CAD build for the part. Positions are in the model's coordinates, mm. A direction names the side the tool comes from. Coordinates: 2 decimals unless noted, no trailing zeros. Order: outer loops, then holes, each group sorted by start corner. A loop starts at its lowest first (then second) coordinate and runs counter-clockwise, first axis right, second up. Notation, with made-up numbers: (37, 68.25) - (75, 68.25) arc R17 ccw to (75, 99.25) - close; hole circle Ø3 at (12.25, -32). An arc over 180 degrees is marked (long way). Return JSON: item names as keys, results as strings.
from build123d import *

# Parameters (mm, degrees)
ESQUISSE1_W             = 80.1
ESQUISSE1_H             = 58.6
BOSS_EXTRU_1_DEPTH      = 19
ESQUISSE2_W             = 12
ESQUISSE2_H             = 58.6
BOSS_EXTRU_2_DEPTH      = 15
ESQUISSE3_R             = 1.25
ENL_V_MAT_EXTRU_1_DEPTH = 105.909341815


with BuildPart() as part:
    # Esquisse1 → Boss.-Extru.1 (new body)
    with BuildSketch(Plane(origin=(0, 0, 0), x_dir=(1, 0, 0), z_dir=(0, 1, 0))):
        with Locations((40.05, 29.3)):
            Rectangle(ESQUISSE1_W, ESQUISSE1_H)
    extrude(amount=BOSS_EXTRU_1_DEPTH)

    # Esquisse2 → Boss.-Extru.2 (add)
    with BuildSketch(Plane.XZ):
        with Locations((43.5, -29.3)):
            Rectangle(ESQUISSE2_W, ESQUISSE2_H)
    extrude(amount=BOSS_EXTRU_2_DEPTH)

    # Esquisse3 → Enlèv. mat.-Extru.1 (cut, through all)
    with BuildSketch(Plane(origin=(0, 19, 0), x_dir=(1, 0, 0), z_dir=(0, 1, 0))):
        with Locations(Location((77.56, 54.79, 0), (0, 0, 270))):
            Circle(ESQUISSE3_R)
        with Locations(Location((25.49, 50.98, 0), (0, 0, 270))):
            Circle(ESQUISSE3_R)
        with Locations(Location((25.49, 1.45, 0), (0, 0, 270))):
            Circle(ESQUISSE3_R)
        with Locations(Location((64.86, 1.45, 0), (0, 0, 270))):
            Circle(ESQUISSE3_R)
    extrude(amount=-ENL_V_MAT_EXTRU_1_DEPTH, mode=Mode.SUBTRACT)


solid = part.part
Item 1: Wall check: L1, parallel to X at y = 12.5, z = -1.45; L2, parallel to Z at x = 64.86, y = 6.25; L3, parallel to X at y = 6.75, z = -50.98. Give the ranges that are in metal, low to high. Write a range as [from, to].
Findings below:
{"L1": "x = [0, 24.24], [26.74, 63.61], [66.11, 80.1]", "L2": "z = [-58.6, -2.7], [-0.2, 0]", "L3": "x = [0, 24.24], [26.74, 80.1]"}
Item 2: Mould opens along X. For faces 4 (the cylindrical face through (65.914, 9.633, -0.778)), 5 (the flat face through (80.1, 9, -29)), 6 (the cylindrical face through (77.61, 9.63, -56.04)), 7 (the flat face through (43, -15, -29)) say: released by +X, released by -X, zero draft, split by the parting line, or undercut.
Findings below:
{"face 4": "undercut", "face 5": "released by +X", "face 6": "undercut", "face 7": "zero draft"}
Item 3: Which spindle directions (+Z, -Z, +X, -X, +Y, -Y) get a long thin tool onto all of the face, cutting with end or side? Do faces 1 (the flat face through (0, 9, -29)), 2 (the flat face through (18, 0, -30)), 3 (the flat face through (65, 0, -30)). Say none if no direction does.
Findings below:
{"face 1": "+Z, -Z, -X, +Y, -Y", "face 2": "+Z, -Z, -X, -Y", "face 3": "+Z, -Z, +X, -Y"}
Item 4: Drop flat-ended pins along their axis: P1, Ø10, axis at y = -7, z = -30, coming from the -X side; P2, Ø4, axis at x = 43, y = -10.5, coming from the +Z side; P3, Ø9, axis at x = 68, z = -43.5, coming from the -Y side; P4, Ø10, axis at y = -6.5, z = -19.5, coming from the +X side. Give the stop position or say it passes through.
Findings below:
{"P1": "stops at x = 37.5", "P2": "stops at z = 0", "P3": "stops at y = 0", "P4": "stops at x = 49.5"}
Item 5: Band-saw the part on C-C, the plane x = 25.49. List the corners of the cut face in (y, z).
Findings below:
{"outline": "(0, -58.6) - (19, -58.6) - (19, -52.23) - (0, -52.23) - close; (0, -49.73) - (19, -49.73) - (19, -2.7) - (0, -2.7) - close; (0, -0.2) - (19, -0.2) - (19, 0) - (0, 0) - close"}
Item 6: Band-saw the part on A-A, the plane x = 77.56. List the corners of the cut face in (y, z), then the cut area to 3 significant figures.
Findings below:
{"outline": "(0, -58.6) - (19, -58.6) - (19, -56.04) - (0, -56.04) - close; (0, -53.54) - (19, -53.54) - (19, 0) - (0, 0) - close", "area": "1,070 mm²"}
Item 7: Band-saw the part on D-D, the plane z = -1.45. List the corners of the cut face in (x, y).
Findings below:
{"outline": "(0, 0) - (24.24, 0) - (24.24, 19) - (0, 19) - close; (26.74, 0) - (37.5, 0) - (37.5, -15) - (49.5, -15) - (49.5, 0) - (63.61, 0) - (63.61, 19) - (26.74, 19) - close; (66.11, 0) - (80.1, 0) - (80.1, 19) - (66.11, 19) - close"}
Item 8: Band-saw the part on B-B, the plane z = -54.79. List the corners of the cut face in (x, y).
Findings below:
{"outline": "(0, 0) - (37.5, 0) - (37.5, -15) - (49.5, -15) - (49.5, 0) - (76.31, 0) - (76.31, 19) - (0, 19) - close; (78.81, 0) - (80.1, 0) - (80.1, 19) - (78.81, 19) - close"}
